Read the model definition and answer for the solid it produces. Units are mm, in the model's axes. Face numbers are marked on the shaded views. A direction names the side the tool comes from. Round coordinates to 2 decimals unless told otherwise and drop trailing zeros. Order: outer loops, then holes, each group sorted by start corner. A loop starts at its lowest first (then second) coordinate and runs counter-clockwise, first axis right, second up. Notation, with made-up numbers: (-28.5, 7.5) -> (23.5, 7.5) arc R7 ccw to (23.5, 14.5) -> close; hole circle Ø5 at (-30.75, 79.25). An arc over 180 degrees is marked (long way). Use a Markdown table: item, result. Add a question column.
1. For the marked faces 1, 2, 3 and 4, determine the directions among +Z, -Z, +X, -X, +Y, -Y from which every point of the face is accessible in a straight line to the end or side of a thin tool.
2. Section D-D, the plane z = 37.5 is taken. Give the vertices of the cut face in (x, y), then the cut area to 3 significant figures.
3. Section C-C, the plane x = -10.5 is taken. Give the vertices of the cut face in (y, z), then the cut area to 3 significant figures.
4. Section A-A, the plane x = 0 is taken. Give the vertices of the cut face in (y, z).
5. Given pin 1 (4 mm diameter, centred on y = -6.5, z = 29, fed in from -X); pin 2 (6 mm diameter, centred on y = 8, z = 8.5, fed in from -X); pin 3 (3 mm diameter, centred on x = 9, z = 43, fed in from +Y), each flat-ended and moving along its own axis, determine where each tip first touches the part or whether it passes through.
6. Consider L1, parallel to Z at x = -8, y = -8.75; L2, parallel to Y at x = -0.25, z = 14; L3, parallel to X at y = -3.75, z = 18. Determine where each line is inside the solid, lowest interval first. Write a range as [from, to].
```python
from build123d import *

# Parameters (mm, degrees)
SKETCH1_R           = 10
BOSS_EXTRUDE1_DEPTH = 50
BOSS_EXTRUDE2_START = -5
SKETCH2_R           = 12.5
BOSS_EXTRUDE2_DEPTH = 5


with BuildPart() as part:
    # Sketch1 → Boss-Extrude1 (new body)
    with BuildSketch(Plane.XY):
        Circle(SKETCH1_R)
    extrude(amount=BOSS_EXTRUDE1_DEPTH)

    # Sketch2 → Boss-Extrude2 (add)
    with BuildSketch(Plane.XY.offset(50).offset(BOSS_EXTRUDE2_START)):
        Circle(SKETCH2_R)
    boss_extrude2 = extrude(amount=-BOSS_EXTRUDE2_DEPTH)

    # Mirror1: Boss-Extrude2 across plane
    add(boss_extrude2.mirror(Plane.XY.offset(25)))


solid = part.part
```
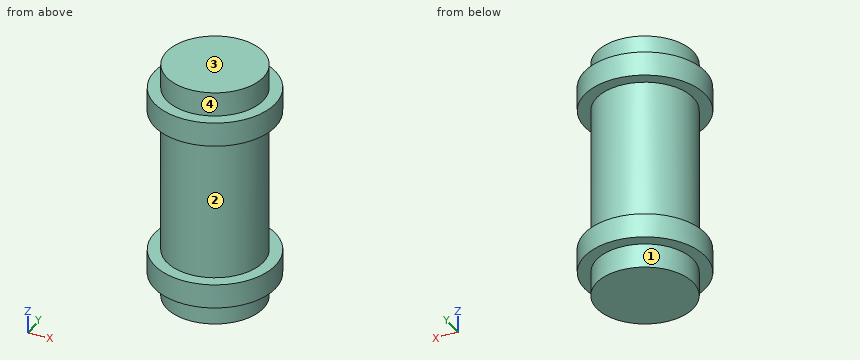
Verdict:
| question | item | result |
|---|---|---|
| 1 | face 1 | -Z |
| 1 | face 2 | none |
| 1 | face 3 | +Z, +X, -X, +Y, -Y |
| 1 | face 4 | +Z |
| 2 | outline | circle Ø20 at (0, 0) |
| 2 | area | 314 mm2 |
| 3 | outline | (-6.78, 5) -> (6.78, 5) -> (6.78, 10) -> (-6.78, 10) -> close; (-6.78, 40) -> (6.78, 40) -> (6.78, 45) -> (-6.78, 45) -> close |
| 3 | area | 136 mm2 |
| 4 | outline | (-12.5, 5) -> (-10, 5) -> (-10, 0) -> (10, 0) -> (10, 5) -> (12.5, 5) -> (12.5, 10) -> (10, 10) -> (10, 40) -> (12.5, 40) -> (12.5, 45) -> (10, 45) -> (10, 50) -> (-10, 50) -> (-10, 45) -> (-12.5, 45) -> (-12.5, 40) -> (-10, 40) -> (-10, 10) -> (-12.5, 10) -> close |
| 5 | pin 1 | stops at x = -8.93 |
| 5 | pin 2 | stops at x = -11.46 |
| 5 | pin 3 | stops at y = 10 |
| 6 | L1 | z = [5, 10], [40, 45] |
| 6 | L2 | y = [-10, 10] |
| 6 | L3 | x = [-9.27, 9.27] |
